from build123d import *

# Parameters (mm, degrees)
SKETCH2_R                       = 3.4925
CUT_EXTRUDE1_DEPTH              = 5.08
SKETCH3_R                       = 12.460238567
CUT_EXTRUDE2_DEPTH              = 3.6576
CUT_EXTRUDE3_DEPTH              = 1.27
CUT_EXTRUDE3_DEPTH_BACK         = 2.54
SKETCH4_R                       = 12.1158
F_4_40_TAPPED_HOLE1_D           = 2.2606
F_4_40_TAPPED_HOLE1_DEPTH       = 2.54
F_4_40_TAPPED_HOLE1_CSINK_D     = 3.048
F_4_40_TAPPED_HOLE1_CSINK_ANGLE = 90
F_4_40_TAPPED_HOLE1_TIP         = 0.679152758


with BuildPart() as part:
    # Sketch1 → Revolve1 (revolve)
    with BuildSketch(Plane.XY, mode=Mode.PRIVATE) as revolve1_sk:
        Polygon((0, 11.176), (1.55575, 11.176), (1.55575, 0), (4.445, 0), (4.445, -1.524), (8.89, -1.524), (13.589, -5.08), (13.589, -5.842), (13.843, -5.842), (13.843, -20.4724), (13.589, -20.4724), (13.589, -23.0124), (12.7, -26.67), (3.81, -26.67), (3.81, -26.924), (1.55575, -26.924), (1.55575, -28.956), (0, -28.956), align=None)
    revolve(revolve1_sk.sketch.rotate(Axis((0, -28.956, 0), (0, 1, 0)), 90), axis=Axis((0, -28.956, 0), (0, 1, 0)))

    # Sketch2 → Cut-Extrude1 (cut)
    with BuildSketch(Plane(origin=(0, -1.524, 0), x_dir=(1, 0, 0), z_dir=(0, 1, 0))):
        with Locations(Location((0, 7.9375, 0), (0, 0, 270))):
            Circle(SKETCH2_R)
        with Locations(Location((7.9375, 0, 0), (0, 0, 270))):
            Circle(SKETCH2_R)
        with Locations(Location((0, -7.9375, 0), (0, 0, 270))):
            Circle(SKETCH2_R)
        with Locations(Location((-7.9375, 0, 0), (0, 0, 270))):
            Circle(SKETCH2_R)
    extrude(amount=-CUT_EXTRUDE1_DEPTH, mode=Mode.SUBTRACT)

    # Sketch3 → Cut-Extrude2 (cut)
    with BuildSketch(Plane.XZ.offset(26.67)):
        with Locations((0, 20.486638567)):
            Circle(SKETCH3_R)
        with Locations((-20.486638567, 0)):
            Circle(SKETCH3_R)
        with Locations((0, -20.486638567)):
            Circle(SKETCH3_R)
        with Locations((20.486638567, 0)):
            Circle(SKETCH3_R)
    extrude(amount=-CUT_EXTRUDE2_DEPTH, mode=Mode.SUBTRACT)

    # Sketch4 → Cut-Extrude3 (cut, two sides: drawn at the far end of the back side and taken through both)
    with BuildSketch(Plane.XZ.offset(23.0124).offset(-CUT_EXTRUDE3_DEPTH_BACK)):
        with Locations(Location((0, 0, 0), (0, 0, 124.065321666))):
            Circle(SKETCH4_R)
    extrude(amount=CUT_EXTRUDE3_DEPTH + CUT_EXTRUDE3_DEPTH_BACK, mode=Mode.SUBTRACT)

    # #4-40 Tapped Hole1
    with Locations(Plane(origin=(0, -26.67, 0), x_dir=(-1, 0, 0), z_dir=(0, -1, 0))):
        with Locations((5.666541612, -5.666541612), (-6.672330298, -6.672330298), (-5.666541612, 5.666541612), (6.672330298, 6.672330298)):
            CounterSinkHole(F_4_40_TAPPED_HOLE1_D / 2, F_4_40_TAPPED_HOLE1_CSINK_D / 2, depth=F_4_40_TAPPED_HOLE1_DEPTH, counter_sink_angle=F_4_40_TAPPED_HOLE1_CSINK_ANGLE)
            with Locations((0, 0, -(F_4_40_TAPPED_HOLE1_DEPTH + F_4_40_TAPPED_HOLE1_TIP / 2))):  # 118° drill point
                Cone(0, F_4_40_TAPPED_HOLE1_D / 2, F_4_40_TAPPED_HOLE1_TIP, mode=Mode.SUBTRACT)


solid = part.part
Build history of the part. All positions in model axes, mm. A direction names the side the tool comes from. Coordinates: 2 decimals unless noted, no trailing zeros. Write each loop counter-clockwise with the first axis right and the second up, starting at its lowest first coordinate (ties: lowest second). Pieces come first, ordered by that corner, then holes. Notation, with made-up numbers: (44.25, 59) -> (77.25, 59) arc R5 cw to (77.25, 65) -> close; hole circle Ø3 at (-8.75, 23). An arc over 180 degrees is marked (long way). Use CSV: the item, a comma, the result in double quotes. Start each with the question number.
Q1. Cut at B-B, the plane y = -1. List the corners of the cut face in (x, z) (3 decimals).
Q2. Drill centre lines: probe 1 along Y at (x, z) = (5, -3.5); probe 2 along Z at (x, y) = (-1.25, -6); probe 3 along X at (y, z) = (-21.7, 0). Where is each one in solid material? Low to high.
Q3. 3-axis set-ups, long thin cutter, end or side, ignore diameter. For faces 1 (the cylindrical face through (-4.08, -21.76, -12.96)), 2 (the cylindrical face through (-4.475, -4.028, -0.455)), 3 (the flat face through (-5, -1.524, -5)): which of +Z, -Z, +X, -X, +Y, -Y reach the whole face in a straight line?
Q4. Flat gauge pins, fed straight in: pin 1 Ø10 at (x, z) = (-3.5, 4) entering from +Y; pin 2 Ø4 at (x, z) = (-2, 4) entering from +Y; pin 3 Ø2 at (x, z) = (-0.5, -9.5) entering from +Y; pin 4 Ø4 at (x, z) = (0, 12.5) entering from -Y. Where does each tip first touch, or does it go through?
Q5. Pull direction X, two halves, no side cores. Call faces 4 (the flat face through (8, -6.604, 0)), 5 (the cylindrical face through (1.38, 5.51, -0.72)), 6 (the conical face through (-9.31, -24.87, 9.27)), 7 (the cylindrical face through (-0.122, -25.273, 8.027)): released by +X, released by -X, zero draft, split by the parting line, or undercut.
Q6. Cut at A-A, the plane y = -12. List the corners of the cut face in (x, z), then the cut area to 3 significant figures.
Checked values:
1,outline,"circle Ø8.89 at (0, 0)"
2,probe 1,"y = -26.67 to -24.28, -20.47 to -1.52"
2,probe 2,"z = -13.79 to -11.2, -4.68 to 4.68, 11.2 to 13.79"
2,probe 3,"x = -13.59 to -12.12, 12.12 to 13.59"
3,face 1,"-Y"
3,face 2,"+Y"
3,face 3,"-Z, -X, +Y"
4,pin 1,"stops at y = 11.18"
4,pin 2,"stops at y = 0"
4,pin 3,"stops at y = -6.6"
4,pin 4,"stops at y = -23.01"
5,face 4,"undercut"
5,face 5,"split by the parting line"
5,face 6,"released by -X"
5,face 7,"undercut"
6,outline,"circle Ø27.69 at (0, 0)"
6,area,"602 mm²"
